For this review, take the finished solid that the model builds, in its own axes (mm). A direction names the side the tool comes from. Round coordinates to 2 decimals unless told otherwise and drop trailing zeros. Loops run counter-clockwise (first coordinate to the right, second up) from the corner with the lowest first, then second, coordinate; pieces in that order, holes last.
1. Tool access review of faces 1 (the cylindrical face through (-9.73, 44.71, 23.87)), 2 (the flat face through (-36.064, 30.859, 10.018)), 3 (the cylindrical face through (-9.069, -14.165, 23.872)): name each direction out of +Z, -Z, +X, -X, +Y, -Y from which nothing blocks a thin tool from reaching the whole face with its end or side.
2. To check wall thickness, follow line 1 along Z through (x, y) = (-16.5, 41.5); line 2 along Y through (x, z) = (-22.5, 13.75); line 3 along Y through (x, z) = (2.5, 5.5). State the ranges of each line that lie inside material, in increasing order.
3. Consider section A-A on z = 11. State the section outline as (x, y) points, then the cut area to 3 significant figures.
4. Consider section B-B on z = 23.5. State the section outline as (x, y) points, then the cut area to 3 significant figures.
5. Clearance check with flat-ended pins moving along their axes: pin 1 Ø12 at (x, z) = (-10, 21) entering from +Y; pin 2 Ø5 at (y, z) = (26.5, 4.5) entering from +X; pin 3 Ø12 at (x, z) = (14, 14.5) entering from -Y. State where each tip first meets the part, or that it passes through.
from build123d import *

# Parameters (mm, degrees)
F1_DEPTH = 25.4
F2_R     = 5.08


with BuildPart() as f1:
    # F0 (on Top) → F1 (new body)
    with BuildSketch(Plane.XY):
        Polygon((-27.146846, -15.661945), (8.517105, -15.565745), (26.265768, 15.368244), (8.35048, 46.206031), (-27.313471, 46.10983), (-45.062134, 15.175842), align=None)
    extrude(amount=F1_DEPTH)

    # F2
    f2_edges = [f1.edges().sort_by_distance(p)[0] for p in [
        (-36.187802, 30.642836, 25.4),
        (-9.481495, 46.15793, 25.4),
        (17.308124, 30.787137, 25.4),
        (17.391437, -0.098751, 25.4),
        (-9.31487, -15.613845, 25.4),
        (-36.10449, -0.243052, 25.4),
    ]]
    fillet(f2_edges, radius=F2_R)


solid = f1.part
Resolved:
1. face 1: +Z, -X, +Y
1. face 2: +Z, -Z, -X, +Y
1. face 3: +Z, +X, -Y
2. line 1: z = 0 to 25.38
2. line 2: y = -15.65 to 46.12
2. line 3: y = -15.58 to 46.19
3. outline: (-45.06, 15.18) - (-27.15, -15.66) - (8.52, -15.57) - (26.27, 15.37) - (8.35, 46.21) - (-27.31, 46.11) - close
3. area: 3,300 mm2
4. outline: (-43.77, 15.18) - (-26.5, -14.54) - (7.87, -14.45) - (24.97, 15.36) - (7.71, 45.09) - (-26.66, 44.99) - close
4. area: 3,070 mm2
5. pin 1: stops at y = 46.17
5. pin 2: stops at x = 21.25
5. pin 3: stops at y = -15.57
